Part model, mm, in its own coordinate system. Face numbers are marked on the shaded views. Round coordinates to 2 decimals unless told otherwise and drop trailing zeros. Write each loop counter-clockwise with the first axis right and the second up, starting at its lowest first coordinate (ties: lowest second). Pieces come first, ordered by that corner, then holes. Notation, with made-up numbers: M -27.5,-2.75 L -14.5,-2.75 A18 cw -14.5,17.25 Z; hole C 74,20 d6. An arc over 180 degrees is marked long. One line per question, with ' | ' between items. Start each with the question number.
1) Mould opens along X. For the marked faces 1, 2, 3 and 4 say: pulls with the +X half, pulls with the -X half, needs draft (parallel to the pull), parting line crosses it, or undercut.
2) Drop flat-ended pins along their axis: pin 1 Ø1.5 at (x, z) = (12.5, 16) entering from -Y; pin 2 Ø1.5 at (x, y) = (18.5, 6.5) entering from +Z. Give the stop position or say it passes through.
3) Saw through at A-A (z = 6). List the corners of the cut face in (x, y).
4) Saw through at C-C (x = -19). List the corners of the cut face in (y, z).
5) Wall check: probe 1 along X at (y, z) = (10.25, -27); probe 2 along Y at (x, z) = (3.5, -19); probe 3 along Z at (x, y) = (22, 7.5). Give the ranges that are in metal, low to high. Write a range as [from, to].
6) Saw through at B-B (y = 22.25). List the corners of the cut face in (x, z), plus the area to 3 significant figures.
```python
from build123d import *

# Parameters (mm, degrees)
ESQUISSE1_W                  = 60
ESQUISSE1_H                  = 150
BOSS_EXTRU_1_DEPTH           = 30
ESQUISSE2_W                  = 50
ESQUISSE2_H                  = 20
ENL_V_MAT_EXTRU_1_DEPTH      = 75
ENL_V_MAT_EXTRU_1_DEPTH_BACK = 70


with BuildPart() as part:
    # Esquisse1 → Boss.-Extru.1 (new body)
    with BuildSketch(Plane(origin=(0, 0, 0), x_dir=(1, 0, 0), z_dir=(0, 1, 0))):
        Rectangle(ESQUISSE1_W, ESQUISSE1_H)
    extrude(amount=BOSS_EXTRU_1_DEPTH)

    # Esquisse2 → Enlèv. mat.-Extru.1 (cut, two sides)
    with BuildSketch(Plane.XY) as enl_v_mat_extru_1_sk:
        with Locations((0, 15)):
            Rectangle(ESQUISSE2_W, ESQUISSE2_H)
    extrude(amount=ENL_V_MAT_EXTRU_1_DEPTH, mode=Mode.SUBTRACT)
    extrude(enl_v_mat_extru_1_sk.sketch, amount=-ENL_V_MAT_EXTRU_1_DEPTH_BACK, mode=Mode.SUBTRACT)


solid = part.part
```
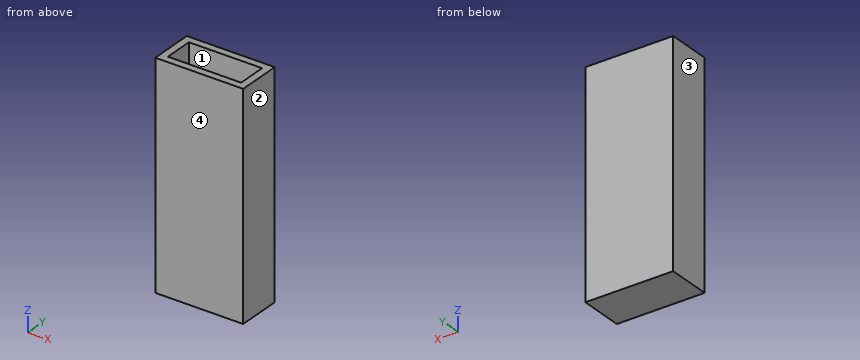
Answer key:
1) face 1: undercut | face 2: pulls with the +X half | face 3: pulls with the -X half | face 4: needs draft
2) pin 1: stops at y = 0 | pin 2: stops at z = -70
3) outline: M -30,0 L 30,0 L 30,30 L -30,30 Z; hole M -25,5 L 25,5 L 25,25 L -25,25 Z
4) outline: M 0,-75 L 30,-75 L 30,75 L 25,75 L 25,-70 L 5,-70 L 5,75 L 0,75 Z
5) probe 1: x = [-30, -25], [25, 30] | probe 2: y = [0, 5], [25, 30] | probe 3: z = [-75, -70]
6) outline: M -30,-75 L 30,-75 L 30,75 L 25,75 L 25,-70 L -25,-70 L -25,75 L -30,75 Z | area: 1,750 mm2
